Can you work these out from the model? Positions are in its coordinate system, mm. A direction names the side the tool comes from. Round coordinates to 2 decimals unless told otherwise and drop trailing zeros. Write each loop counter-clockwise with the first axis right and the second up, starting at its lowest first coordinate (ties: lowest second). Pieces come first, ordered by that corner, then holes. Notation, with made-up numbers: M 19.5,33.5 L 56.5,33.5 A20 ccw 56.5,41.5 Z; hole C -3,75 d4. An arc over 180 degrees is marked long. Use one line per item in the form item = value. Start each with the question number.
```python
from build123d import *

# Parameters (mm, degrees)
CROQUIS1_R              = 3
SALIENTE_EXTRUIR1_DEPTH = 6


with BuildPart() as part:
    # Croquis1 → Saliente-Extruir1 (new body)
    with BuildSketch(Plane(origin=(0, 0, 0), x_dir=(1, 0, 0), z_dir=(0, 1, 0))):
        with BuildLine():
            Line((39.015376651, -43.078821925), (100.511897923, -43.078821925))
            ThreePointArc((100.511897923, -43.078821925), (107.582965735, -40.149889737), (110.511897923, -33.078821925))
            Line((110.511897923, -33.078821925), (110.511897923, 33.078821925))
            ThreePointArc((110.511897923, 33.078821925), (107.582965735, 40.149889737), (100.511897923, 43.078821925))
            Line((100.511897923, 43.078821925), (39.015376651, 43.078821925))
            ThreePointArc((39.015376651, 43.078821925), (34.772735964, 41.321462613), (33.015376651, 37.078821925))
            Line((33.015376651, 37.078821925), (33.015376651, 33))
            ThreePointArc((33.015376651, 33), (31.258017338, 28.757359313), (27.015376651, 27))
            Line((27.015376651, 27), (-27.015376651, 27))
            ThreePointArc((-27.015376651, 27), (-31.258017338, 28.757359313), (-33.015376651, 33))
            Line((-33.015376651, 33), (-33.015376651, 37.078821925))
            ThreePointArc((-33.015376651, 37.078821925), (-34.772735964, 41.321462613), (-39.015376651, 43.078821925))
            Line((-39.015376651, 43.078821925), (-100.511897923, 43.078821925))
            ThreePointArc((-100.511897923, 43.078821925), (-107.582965735, 40.149889737), (-110.511897923, 33.078821925))
            Line((-110.511897923, 33.078821925), (-110.511897923, -33.078821925))
            ThreePointArc((-110.511897923, -33.078821925), (-107.582965735, -40.149889737), (-100.511897923, -43.078821925))
            Line((-100.511897923, -43.078821925), (-39.015376651, -43.078821925))
            ThreePointArc((-39.015376651, -43.078821925), (-34.772735964, -41.321462613), (-33.015376651, -37.078821925))
            Line((-33.015376651, -37.078821925), (-33.015376651, -33))
            ThreePointArc((-33.015376651, -33), (-31.258017338, -28.757359313), (-27.015376651, -27))
            Line((-27.015376651, -27), (27.015376651, -27))
            ThreePointArc((27.015376651, -27), (31.258017338, -28.757359313), (33.015376651, -33))
            Line((33.015376651, -33), (33.015376651, -37.078821925))
            ThreePointArc((33.015376651, -37.078821925), (34.772735964, -41.321462613), (39.015376651, -43.078821925))
        make_face()
        with BuildLine():
            Line((-100, -25.75), (-79.25, -25.75))
            Line((-79.25, -25.75), (-79.25, -19.25))
            Line((-79.25, -19.25), (-100, -19.25))
            ThreePointArc((-100, -19.25), (-104.25, -15), (-100, -10.75))
            Line((-100, -10.75), (-79.25, -10.75))
            Line((-79.25, -10.75), (-79.25, -4.25))
            Line((-79.25, -4.25), (-100, -4.25))
            ThreePointArc((-100, -4.25), (-104.25, 0), (-100, 4.25))
            Line((-100, 4.25), (-79.25, 4.25))
            Line((-79.25, 4.25), (-79.25, 10.75))
            Line((-79.25, 10.75), (-100, 10.75))
            ThreePointArc((-100, 10.75), (-104.25, 15), (-100, 19.25))
            Line((-100, 19.25), (-79.25, 19.25))
            Line((-79.25, 19.25), (-79.25, 25.75))
            Line((-79.25, 25.75), (-100, 25.75))
            ThreePointArc((-100, 25.75), (-104.25, 30), (-100, 34.25))
            Line((-100, 34.25), (-75, 34.25))
            Line((-75, 34.25), (-50, 34.25))
            ThreePointArc((-50, 34.25), (-45.75, 30), (-50, 25.75))
            Line((-50, 25.75), (-70.75, 25.75))
            Line((-70.75, 25.75), (-70.75, 19.25))
            Line((-70.75, 19.25), (-50, 19.25))
            ThreePointArc((-50, 19.25), (-45.75, 15), (-50, 10.75))
            Line((-50, 10.75), (-70.75, 10.75))
            Line((-70.75, 10.75), (-70.75, 4.25))
            Line((-70.75, 4.25), (-50, 4.25))
            ThreePointArc((-50, 4.25), (-45.75, 0), (-50, -4.25))
            Line((-50, -4.25), (-70.75, -4.25))
            Line((-70.75, -4.25), (-70.75, -10.75))
            Line((-70.75, -10.75), (-50, -10.75))
            ThreePointArc((-50, -10.75), (-45.75, -15), (-50, -19.25))
            Line((-50, -19.25), (-70.75, -19.25))
            Line((-70.75, -19.25), (-70.75, -25.75))
            Line((-70.75, -25.75), (-50, -25.75))
            ThreePointArc((-50, -25.75), (-45.75, -30), (-50, -34.25))
            Line((-50, -34.25), (-75, -34.25))
            Line((-75, -34.25), (-100, -34.25))
            ThreePointArc((-100, -34.25), (-104.25, -30), (-100, -25.75))
        make_face(mode=Mode.SUBTRACT)
        with Locations(Location((0, -17.5, 0), (0, 0, 270))):
            Circle(CROQUIS1_R, mode=Mode.SUBTRACT)
        with BuildLine():
            Line((79.25, -19.25), (79.25, -25.9432425))
            Line((79.25, -25.9432425), (100, -25.9432425))
            ThreePointArc((100, -25.9432425), (104.0567575, -30), (100, -34.0567575))
            Line((100, -34.0567575), (76.266972211, -34.0567575))
            ThreePointArc((76.266972211, -34.0567575), (75, -34.25), (73.733027789, -34.0567575))
            Line((73.733027789, -34.0567575), (50, -34.0567575))
            ThreePointArc((50, -34.0567575), (45.9432425, -30), (50, -25.9432425))
            Line((50, -25.9432425), (70.75, -25.9432425))
            Line((70.75, -25.9432425), (70.75, -19.25))
            Line((70.75, -19.25), (50, -19.25))
            ThreePointArc((50, -19.25), (45.75, -15), (50, -10.75))
            Line((50, -10.75), (70.75, -10.75))
            Line((70.75, -10.75), (70.75, -4.25))
            Line((70.75, -4.25), (50, -4.25))
            ThreePointArc((50, -4.25), (45.75, 0), (50, 4.25))
            Line((50, 4.25), (70.75, 4.25))
            Line((70.75, 4.25), (70.75, 10.75))
            Line((70.75, 10.75), (50, 10.75))
            ThreePointArc((50, 10.75), (45.75, 15), (50, 19.25))
            Line((50, 19.25), (70.75, 19.25))
            Line((70.75, 19.25), (70.75, 26.012157078))
            Line((70.75, 26.012157078), (50, 26.012157078))
            ThreePointArc((50, 26.012157078), (46.012157078, 30), (50, 33.987842922))
            Line((50, 33.987842922), (73.530439238, 33.987842922))
            ThreePointArc((73.530439238, 33.987842922), (75, 34.25), (76.469560762, 33.987842922))
            Line((76.469560762, 33.987842922), (100, 33.987842922))
            ThreePointArc((100, 33.987842922), (103.987842922, 30), (100, 26.012157078))
            Line((100, 26.012157078), (79.25, 26.012157078))
            Line((79.25, 26.012157078), (79.25, 19.25))
            Line((79.25, 19.25), (100, 19.25))
            ThreePointArc((100, 19.25), (104.25, 15), (100, 10.75))
            Line((100, 10.75), (79.25, 10.75))
            Line((79.25, 10.75), (79.25, 4.25))
            Line((79.25, 4.25), (100, 4.25))
            ThreePointArc((100, 4.25), (104.25, 0), (100, -4.25))
            Line((100, -4.25), (79.25, -4.25))
            Line((79.25, -4.25), (79.25, -10.75))
            Line((79.25, -10.75), (100, -10.75))
            ThreePointArc((100, -10.75), (104.25, -15), (100, -19.25))
            Line((100, -19.25), (79.25, -19.25))
        make_face(mode=Mode.SUBTRACT)
        with Locations(Location((0, 17.5, 0), (0, 0, 270))):
            Circle(CROQUIS1_R, mode=Mode.SUBTRACT)
    extrude(amount=SALIENTE_EXTRUIR1_DEPTH)


solid = part.part
```
1. If we section it at D-D (y = 4.85): State how many separate pieces and enclosed holes the cut face has, and give its area (3 significant figures).
2. Please list where these lines run through material, in increasing order: line 1 along Z through (x, y) = (69.5, 1.75); line 2 along X through (y, z) = (0.3, 3); line 3 along X through (y, z) = (3.9, -29).
3. If we section it at C-C (x = 84): List the corners of the cut face in (y, z) for me.
4. If we section it at B-B (x = -73.5): List the corners of the cut face in (y, z) for me, and give its area (3 significant figures).
5. Will these pins go through, and if not, where does the flat tip stop? pin 1 (2 mm diameter, centred on x = -9.5, y = 3, fed in from +Z); pin 2 (2 mm diameter, centred on x = -1.5, y = 2.5, fed in from -Z).
6. Which directions (+Z, -Z, +X, -X, +Y, -Y) give clear straight access to the entire face, cutting with the end or side of a thin tool? Please do faces 1 (the face through (-31.2, 3, -28.7)), 2 (the face through (-60, 3, -10.75)).
7. If we mould it in two halves opening along X, with no side actions, what happens to faces 3 (the face through (-45.75, 2.96, -30.09)), 4 (the face through (-104.25, 2.96, -14.91)), 5 (the face through (110.512, 3, 0))? For each: pulls with the +X half, pulls with the -X half, needs draft (parallel to the pull), parting line crosses it, or undercut.
8. If we section it at A-A (x = 0): List the corners of the cut face in (y, z) for me.
Model answer:
q1.separate_pieces = 1
q1.enclosed_holes = 4
q1.area = 11,600 mm2
q2.line_1 = -43.08 to -33.99, -26.01 to -19.25, -10.75 to -4.25, 4.25 to 10.75, 19.25 to 25.94, 34.06 to 43.08
q2.line_2 = -110.51 to -103.01, -46.99 to 46.99, 103.01 to 110.51
q2.line_3 = -110.51 to -104.13, -45.87 to -31.49, 31.49 to 46.14, 103.86 to 110.51
q3.outline = M 0,-43.08 L 6,-43.08 L 6,-33.99 L 0,-33.99 Z; M 0,-26.01 L 6,-26.01 L 6,-19.25 L 0,-19.25 Z; M 0,-10.75 L 6,-10.75 L 6,-4.25 L 0,-4.25 Z; M 0,4.25 L 6,4.25 L 6,10.75 L 0,10.75 Z; M 0,19.25 L 6,19.25 L 6,25.94 L 0,25.94 Z; M 0,34.06 L 6,34.06 L 6,43.08 L 0,43.08 Z
q4.outline = M 0,-43.08 L 6,-43.08 L 6,-34.25 L 0,-34.25 Z; M 0,34.25 L 6,34.25 L 6,43.08 L 0,43.08 Z
q4.area = 106 mm2
q5.pin_1 = 27
q5.pin_2 = -27
q6.face_1 = -Z, +Y, -Y
q6.face_2 = +Y, -Y
q7.face_3 = undercut
q7.face_4 = undercut
q7.face_5 = pulls with the +X half
q8.outline = M 0,-27 L 6,-27 L 6,-20.5 L 0,-20.5 Z; M 0,-14.5 L 6,-14.5 L 6,14.5 L 0,14.5 Z; M 0,20.5 L 6,20.5 L 6,27 L 0,27 Z
